The listing builds one solid part. Answer for the finished solid, in the listing's coordinates (mm). Give positions to 0.01 mm unless a question says otherwise; leave off trailing zeros. Write each loop counter-clockwise with the first axis right and the second up, starting at its lowest first coordinate (ties: lowest second). Pieces come first, ordered by that corner, then holes.
```python
from build123d import *

# Parameters (mm, degrees)
F0_R     = 11
F2_R     = 8
F4_R     = 3
F5_R     = 0.5
F6_DEPTH = 20


with BuildPart() as f3:
    # F0 (on Top) → F3 section 0
    with BuildSketch(Plane.XY):
        Circle(F0_R)
    # F2 (on offset) → F3 section 1
    with BuildSketch(Plane.XY.offset(-20)):
        Circle(F2_R)
    loft()

    # F4
    f4_edges = [f3.edges().sort_by_distance(p)[0] for p in [
        (-8, 0, -20),
    ]]
    fillet(f4_edges, radius=F4_R)

    # F5 (on face) → F6 (cut)
    with BuildSketch(Plane(origin=(0, 0, -20), x_dir=(1, 0, 0), z_dir=(0, 0, -1))):
        Circle(F5_R)
    extrude(amount=-F6_DEPTH, mode=Mode.SUBTRACT)


solid = f3.part
```
Item 1: Determine the mould class of faces 1 (the face through (8.95, 2.82, -10.78)), 2 (the face through (0, -2, 0)), 3 (the face through (-0.108, 0.488, -10.14)) for opening direction X: pulls with the +X half, pulls with the -X half, needs draft (parallel to the pull), parting line crosses it, or undercut.
Conclusion:
face 1: parting line crosses it
face 2: needs draft
face 3: undercut
Item 2: A cutting plane is placed at C-C, the plane z = -12.5. Give the vertices of the cut face in (x, y) (3 decimals), plus the area to 3 significant figures.
Conclusion:
outline: circle Ø18.25 at (0, 0); hole circle Ø1 at (0, 0)
area: 261 mm2
Item 3: Consider probe 1 along Z at (x, y) = (4.25, 3.5); probe 2 along Y at (x, z) = (0, -8.75); probe 3 along X at (y, z) = (0, -13.25). Determine where each line is inside the solid, lowest interval first.
Conclusion:
probe 1: z = -20 to 0
probe 2: y = -9.69 to -0.5, 0.5 to 9.69
probe 3: x = -9.01 to -0.5, 0.5 to 9.01
Item 4: Each of these flat-tipped pins is pushed along its axis until it touches: P1, Ø6, axis at x = 3.5, z = -6.5, coming from the -Y side; P2, Ø1.5, axis at x = -5.5, z = -4.5, coming from the +Y side; P3, Ø3, axis at x = 5.5, z = -13, coming from the -Y side. Where does it stop, or does it pass through?
Conclusion:
P1: stops at y = -10.25
P2: stops at y = 9.19
P3: stops at y = -8.16
Item 5: A cutting plane is placed at B-B, the plane z = -7. Give the vertices of the cut face in (x, y), plus the area to 3 significant figures.
Conclusion:
outline: circle Ø19.9 at (0, 0); hole circle Ø1 at (0, 0)
area: 310 mm2
Item 6: A cutting plane is placed at A-A, the plane x = 0. Give the vertices of the cut face in (y, z).
Conclusion:
outline: (-11, 0) - (-8.38, -17.45) arc R3 ccw to (-5.42, -20) - (-0.5, -20) - (-0.5, 0) - close; (0.5, -20) - (5.42, -20) arc R3 ccw to (8.38, -17.45) - (11, 0) - (0.5, 0) - close
